Could you check a few things on this model? Use its own coordinates, in mm. A direction names the side the tool comes from. Round coordinates to 2 decimals unless told otherwise and drop trailing zeros. Write each loop counter-clockwise with the first axis right and the second up, starting at its lowest first coordinate (ties: lowest second). Pieces come first, ordered by that corner, then holes. Notation, with made-up numbers: (49, -22.75) -> (105, -22.75) arc R29 ccw to (105, 15.25) -> close; hole circle Ø7 at (-29, 42). An arc over 180 degrees is marked (long way). One line per question, with ' | ' between items. Start each with the question number.
1. Imagine slicing it at C-C, the plane y = -1. State how many separate pieces and enclosed holes the cut face has, and give its area (3 significant figures).
2. Imagine slicing it at B-B, the plane x = 0. List the corners of the cut face in (y, z) for me (3 decimals).
3. If I drill on line 1 along X through (y, z) = (0, 5.5) (3 decimals); line 2 along Z through (x, y) = (-0.75, -2.5); line 3 along X through (y, z) = (3.1, 6.95), over which ranges is the centre line in solid material (lowest first)? Write a range as [from, to].
4. For faces 1 (the flat face through (1, -2.2, 6.3)), 2 (the flat face through (0, 1.2, 4)), 3 (the cylindrical face through (2.25, 3.07, 7.18)), which set-ups out of +Z, -Z, +X, -X, +Y, -Y let a thin tool reach every point of the face, with its end or its side?
5. Thinking about a two-plate mould opening in X: for faces 4 (the flat face through (-2.2, 1, 1.5)), 5 (the flat face through (0, 2, 0)), which applies, released by +X, released by -X, zero draft, split by the parting line, or undercut?
6. For pin 1 Ø2 at (y, z) = (2, 5.5) entering from +X; pin 2 Ø3 at (y, z) = (4, 3.5) entering from -X, each with a flat end and sliding along its axis, tell me the tip position at first contact or that it passes through.
7. Imagine slicing it at A-A, the plane z = 2.5. List the corners of the cut face in (x, y) for me (3 decimals), and give its area (3 significant figures).
Solid Edge part; units mm, degrees
sketch "Sketch1" plane through (0, 0, 0) normal (0, -1, 0) x (1, 0, 0)
  line L0 (5, 6.3) -> (2.25, 6.3)
  line L1 (2.25, 6.3) -> (2.25, 1.5)
  line L2 (5, 1.5) -> (2.25, 1.5)
  line L3 (5, 0) -> (5, 1.5)
  line L4 (0, 0) -> (5, 0)
  line L5 (0, 7.8) -> (0, 0)
  line L6 (5, 7.8) -> (0, 7.8)
  line L7 (5, 7.8) -> (5, 6.3)
revolve "RevolvedProtrusion1" add sketch "Sketch1" angle 360 about axis through (0, 0, 7.8) along (0, 0, -1)
sketch "Sketch2" plane through (0, 0, 7.8) normal (0, 0, 1) x (1, 0, 0)
  line L0 (-1.0957, 1.2) -> (1.0957, 1.2)
  arc A0 (1.0957, 1.2) -> (-1.0957, 1.2) centre (0, 0) cw
extrude "Cutout1" cut sketch "Sketch2" against normal through all
sketch "Sketch3" plane through (0, 0, 7.8) normal (0, 0, 1) x (-1, 0, 0)
  circle A0 centre (-1.5, -3.1) radius 0.75
  circle A1 centre (1.5, -3.1) radius 0.75
extrude "Cutout2" cut sketch "Sketch3" against normal up to surface (1.5 mm away)
chamfer "Chaflán_1" distance 0.25 angle 45 4 edges at (-5, 0, 0) (-5, 0, 1.5) (-5, 0, 6.3) (-5, 0, 7.8)
sketch "Sketch4" plane through (0, 0, 0) normal (1, 0, 0) x (0, 1, 0)
  circle A0 centre (3.1, 7.8) radius 0.75
extrude "VaciadoExtruido_3" cut sketch "Sketch4" along normal mid plane 3
fillet "Redondeo_2" radius 0.5 2 edges at (-0.75, 3.1, 7.05) (0.75, 3.1, 7.05)
fillet "Redondeo_3" radius 0.25 2 edges at (2.25, 3.1, 6.3) (-0.75, 3.1, 6.3)
sketch "Sketch5" plane through (0, 0, 1.5) normal (0, 0, 1) x (0, 1, 0)
  circle A0 centre (0, 0) radius 5
  circle A1 centre (0, 0) radius 4.75
extrude "ProtrusiónExtruida_1" add sketch "Sketch5" against normal blind 0.25 and the other way up to vertex (5.05 mm away)
Geometry results:
1) separate pieces: 2 | enclosed holes: 2 | area: 31.1 mm2
2) outline: (-5, 0.25) -> (-4.75, 0) -> (-1.625, 0) -> (-1.625, 7.8) -> (-4.75, 7.8) -> (-5, 7.55) -> close; (1.2, 0) -> (4.75, 0) -> (5, 0.25) -> (5, 7.55) -> (4.75, 7.8) -> (3.85, 7.8) arc R0.75 cw to (2.35, 7.8) -> (1.2, 7.8) -> close; hole (-4.75, 1.5) -> (-2.25, 1.5) -> (-2.25, 6.3) -> (-4.75, 6.3) -> close; hole (2.25, 1.5) -> (4.75, 1.5) -> (4.75, 6.3) -> (2.25, 6.3) -> close
3) line 1: x = [-5, -4.75], [-2.25, -1.625], [1.625, 2.25], [4.75, 5] | line 2: z = [0, 1.5], [6.3, 7.8] | line 3: x = [-3.92, -2.25], [-0.55, 0.55], [2.25, 3.92]
4) face 1: none | face 2: +Z, -Z | face 3: +Z
5) face 4: undercut | face 5: zero draft
6) pin 1: stops at x = 4.9 | pin 2: stops at x = -4.33
7) outline: circle Ø10 at (0, 0); circle Ø4.5 at (0, 0); hole circle Ø9.5 at (0, 0); hole (-1.096, 1.2) arc R1.625 ccw (long way) to (1.096, 1.2) -> close | area: 15.9 mm2
